from build123d import *

# Parameters (mm, degrees)
SKETCH_1_R          = 1.8
SKETCH_1_R_2        = 1.225
EXTRUDE_1_DEPTH     = 7
SKETCH_2_W          = 0.5
SKETCH_2_H          = 2.37615298
CUT_EXTRUDE_1_DEPTH = 8.44848978


with BuildPart() as part:
    # 草图1 → 凸台-拉伸1 (new body)
    with BuildSketch(Plane(origin=(0, 0, 0), x_dir=(1, 0, 0), z_dir=(0, 1, 0))):
        with Locations(Location((0, 0, 0), (0, 0, 270))):
            Circle(SKETCH_1_R)
        with Locations(Location((0, 0, 0), (0, 0, 270))):
            Circle(SKETCH_1_R_2, mode=Mode.SUBTRACT)
    extrude(amount=EXTRUDE_1_DEPTH)

    # 草图2 → 切除-拉伸1 (cut, through all)
    with BuildSketch(Plane(origin=(0, 7, 0), x_dir=(1, 0, 0), z_dir=(0, 1, 0))):
        with Locations((0, 1.8)):
            Rectangle(SKETCH_2_W, SKETCH_2_H)
    extrude(amount=-CUT_EXTRUDE_1_DEPTH, mode=Mode.SUBTRACT)


solid = part.part
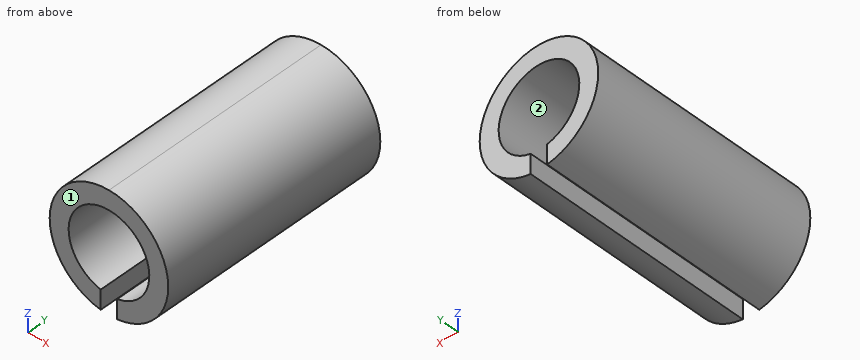
The listing builds one solid part. Answer for the finished solid, in the listing's coordinates (mm). Face numbers are marked on the shaded views. Give positions to 0.01 mm unless a question says otherwise; leave off trailing zeros. Loops run counter-clockwise (first coordinate to the right, second up) from the corner with the lowest first, then second, coordinate; pieces in that order, holes last. Notation, with made-up numbers: (0, 49.25) - (34, 49.25) arc R14 cw to (34, 60.25) - close; hole circle Ø3 at (30, 74.5). An arc over 180 degrees is marked (long way). Answer as a JSON object with one key per item and string values.
1. Find the intervals of material crossed by L1, parallel to X at y = 2, z = 0 (3 decimals); L2, parallel to Z at x = 0, y = 2.75 (3 decimals); L3, parallel to X at y = 6.25, z = -0.75, in increasing order. Write a range as [from, to].
Determined:
{"L1": "[-1.8, -1.225], [1.225, 1.8]", "L2": "[1.225, 1.8]", "L3": "[-1.64, -0.97], [0.97, 1.64]"}
2. A cutting plane is placed at B-B (x = 0.7). Write down the section's boundary in (y, z).
Determined:
{"outline": "(0, -1.66) - (7, -1.66) - (7, -1.01) - (0, -1.01) - close; (0, 1.01) - (7, 1.01) - (7, 1.66) - (0, 1.66) - close"}
3. A cutting plane is placed at D-D (z = 1.35). Write down the section's boundary in (x, y).
Determined:
{"outline": "(-1.19, 0) - (1.19, 0) - (1.19, 7) - (-1.19, 7) - close"}
4. A cutting plane is placed at C-C (y = 5.5). Write down the section's boundary in (x, z) (3 decimals).
Determined:
{"outline": "(-0.25, -1.783) - (-0.25, -1.199) arc R1.225 cw (long way) to (0.25, -1.199) - (0.25, -1.783) arc R1.8 ccw (long way) to start"}
5. For a pull along Z with two mould halves and no side action, classify the marked faces 1 and 2 as pulls with the +Z half, pulls with the -Z half, needs draft (parallel to the pull), parting line crosses it, or undercut.
Determined:
{"face 1": "needs draft", "face 2": "undercut"}
6. A flat-ended cylindrical pin translates along its axis: pin 1 Ø2 at (x, z) = (0, 0) entering from +Y. Find the tip coordinate at first contact, or state that the pin passes through.
Determined:
{"pin 1": "through"}
7. A cutting plane is placed at A-A (z = 0). Write down the section's boundary in (x, y) (3 decimals).
Determined:
{"outline": "(-1.8, 0) - (-1.225, 0) - (-1.225, 7) - (-1.8, 7) - close; (1.225, 0) - (1.8, 0) - (1.8, 7) - (1.225, 7) - close"}
